Job drawing, mm, ordinate dimensions from the low corner. One solid piece. Give positions to 0.01 mm unless a question says otherwise; leave off trailing zeros. Order: outer loops, then holes, each group sorted by start corner. A loop starts at its lowest first (then second) coordinate and runs counter-clockwise, first axis right, second up.
Item 1: Band-saw the part on D-D on x = 24.5. Give the cut face in (y, z).
Item 2: Wall check: L1, parallel to X at y = 1.2, z = 5; L2, parallel to Z at x = 15.25, y = 2.8; L3, parallel to X at y = 1, z = 25. Give the ranges that are in metal, low to high.
Item 3: Band-saw the part on A-A on x = 15. Give the cut face in (y, z), plus the area to 3 significant figures.
Item 4: Band-saw the part on B-B on z = 25. Give the cut face in (x, y).
Item 5: Flat gauge pin, fed straight in: P1, Ø1.5, axis at y = 2, z = 6, coming from the -X side. Where does the tip first touch, or does it go through?
Item 6: Band-saw the part on C-C on y = 1.25. Give the cut face in (x, z), plus the area to 3 significant figures.
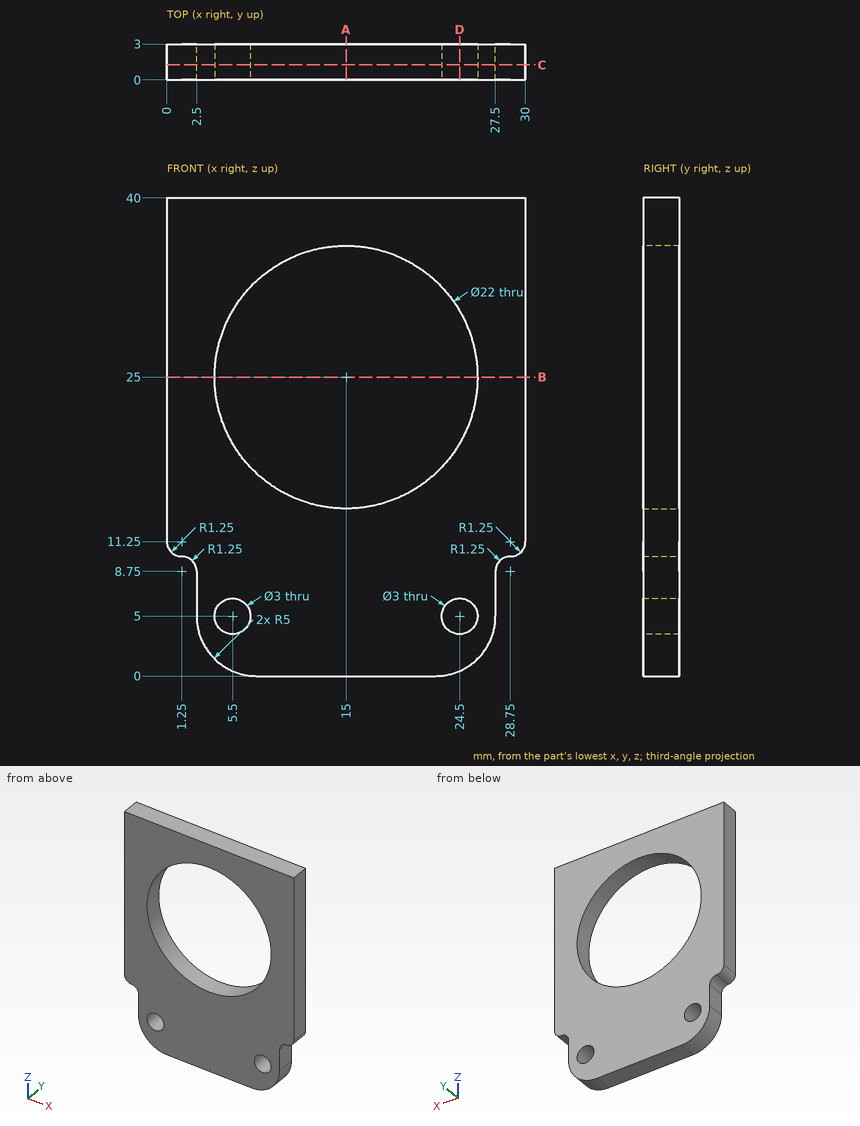
The answers:
1. outline: (0, 0.42) - (3, 0.42) - (3, 3.5) - (0, 3.5) - close; (0, 6.5) - (3, 6.5) - (3, 19.45) - (0, 19.45) - close; (0, 30.55) - (3, 30.55) - (3, 40) - (0, 40) - close
2. L1: x = 2.5 to 4, 7 to 23, 26 to 27.5
2. L2: z = 0 to 14, 36 to 40
2. L3: x = 0 to 4, 26 to 30
3. outline: (0, 0) - (3, 0) - (3, 14) - (0, 14) - close; (0, 36) - (3, 36) - (3, 40) - (0, 40) - close
3. area: 54.0 mm2
4. outline: (0, 0) - (4, 0) - (4, 3) - (0, 3) - close; (26, 0) - (30, 0) - (30, 3) - (26, 3) - close
5. P1: stops at x = 2.5
6. outline: (0, 11.25) arc R1.25 ccw to (1.25, 10) arc R1.25 cw to (2.5, 8.75) - (2.5, 5) arc R5 ccw to (7.5, 0) - (22.5, 0) arc R5 ccw to (27.5, 5) - (27.5, 8.75) arc R1.25 cw to (28.75, 10) arc R1.25 ccw to (30, 11.25) - (30, 40) - (0, 40) - close; hole circle Ø3 at (5.5, 5); hole circle Ø22 at (15, 25); hole circle Ø3 at (24.5, 5)
6. area: 745 mm2
